```python
from build123d import *

# Parameters (mm, degrees)
EXTRUDE_1_DEPTH     = 39
SKETCH_3_R          = 1.65
CUT_EXTRUDE_1_DEPTH = 10
SKETCH_4_R          = 1.65
CUT_EXTRUDE_2_DEPTH = 10


with BuildPart() as part:
    # 草图1 → 凸台-拉伸1 (new body)
    with BuildSketch(Plane.XY):
        Polygon((0, 0), (77.940672381, 0), (102.547661001, 5.230376894), (102.131837619, 7.186672096), (76.7, 1.780968134), (0, 1.780968134), align=None)
    extrude(amount=EXTRUDE_1_DEPTH)

    # 草图3 → 切除-拉伸1 (cut)
    with BuildSketch(Plane(origin=(2.953339199, -13.89436852, 0), x_dir=(0.9781476007338052, 0.20791169081776095, 0), z_dir=(-0.20791169081776098, 0.9781476007338054, 0))):
        with Locations(Location((90.394205072, -11.5, 0), (0, 0, 180))):
            Circle(SKETCH_3_R)
        with Locations(Location((90.394205072, -27.5, 0), (0, 0, 180))):
            Circle(SKETCH_3_R)
    extrude(amount=-CUT_EXTRUDE_1_DEPTH, mode=Mode.SUBTRACT)

    # 草图4 → 切除-拉伸2 (cut)
    with BuildSketch(Plane(origin=(0, 1.780968134, 0), x_dir=(1, 0, 0), z_dir=(0, 1, 0))):
        with Locations(Location((20.25, -5, 0), (0, 0, 180))):
            Circle(SKETCH_4_R)
        with Locations(Location((51.95, -5, 0), (0, 0, 180))):
            Circle(SKETCH_4_R)
        with Locations(Location((51.95, -34, 0), (0, 0, 270))):
            Circle(SKETCH_4_R)
        with Locations(Location((20.25, -34, 0), (0, 0, 270))):
            Circle(SKETCH_4_R)
    extrude(amount=-CUT_EXTRUDE_2_DEPTH, mode=Mode.SUBTRACT)


solid = part.part
```
Can you work these out from the model? Positions are in its coordinate system, mm. A direction names the side the tool comes from. Give positions to 0.01 mm unless a question says otherwise; leave off trailing zeros. Write each loop counter-clockwise with the first axis right and the second up, starting at its lowest first coordinate (ties: lowest second). Pieces come first, ordered by that corner, then holes. Notation, with made-up numbers: (85, 82) -> (120, 82) arc R28 ccw to (120, 106) -> close; hole circle Ø7 at (39.5, -18). An arc over 180 degrees is marked (long way). One line per item, written item: value.
Q1. We'd pull the mould along Z, two halves only. Please class faces 1 (the face through (51, 1, 39)), 2 (the face through (38, 0, 19)), 3 (the face through (91.787, 3.98, 29.136)): +Z half, -Z half, draft (parallel to the pull), parting line (faces both ways), or undercut.
Results found:
face 1: +Z half
face 2: draft
face 3: undercut
Q2. Imagine slicing it at B-B on x = 20.25. Please give me the cut outline in (y, z).
Results found:
outline: (0, 0) -> (1.78, 0) -> (1.78, 3.35) -> (0, 3.35) -> close; (0, 6.65) -> (1.78, 6.65) -> (1.78, 32.35) -> (0, 32.35) -> close; (0, 35.65) -> (1.78, 35.65) -> (1.78, 39) -> (0, 39) -> close
Q3. Imagine slicing it at C-C on z = 19.5. Please give me the cut outline in (x, y).
Results found:
outline: (0, 0) -> (77.94, 0) -> (102.55, 5.23) -> (102.13, 7.19) -> (76.7, 1.78) -> (0, 1.78) -> close
Q4. Imagine slicing it at A-A on z = 34. Please give me the cut outline in (x, y), and give its area (3 significant figures).
Results found:
outline: (0, 0) -> (18.6, 0) -> (18.6, 1.78) -> (0, 1.78) -> close; (21.9, 0) -> (50.3, 0) -> (50.3, 1.78) -> (21.9, 1.78) -> close; (53.6, 0) -> (77.94, 0) -> (102.55, 5.23) -> (102.13, 7.19) -> (76.7, 1.78) -> (53.6, 1.78) -> close
area: 177 mm^2
Q5. For P1, Ø8, axis at x = 69.5, z = 33.5, coming from the +Y side; P2, Ø2, axis at x = 20.25, z = 5, coming from the +Y side; P3, Ø4, axis at y = 1, z = 11, coming from the +X side, each with a flat end and sliding along its axis, tell me the tip position at first contact or that it passes through.
Results found:
P1: stops at y = 1.78
P2: passes through
P3: stops at x = 90.98
Q6. Please list where these lines run through material, in increasing order: line 1 (Z direction, x = 51, y = 0.5); line 2 (Y direction, x = 71.5, z = 14). Write a range as [from, to].
Results found:
line 1: z = [0, 3.65], [6.35, 32.65], [35.35, 39]
line 2: y = [0, 1.78]
Q7. Which directions (+Z, -Z, +X, -X, +Y, -Y) give clear straight access to the entire face, cutting with the end or side of a thin tool? Please do faces 4 (the face through (39, 1.781, 19)), 5 (the face through (0, 1, 19)).
Results found:
face 4: +Z, -Z, -X, +Y
face 5: +Z, -Z, -X, +Y, -Y
